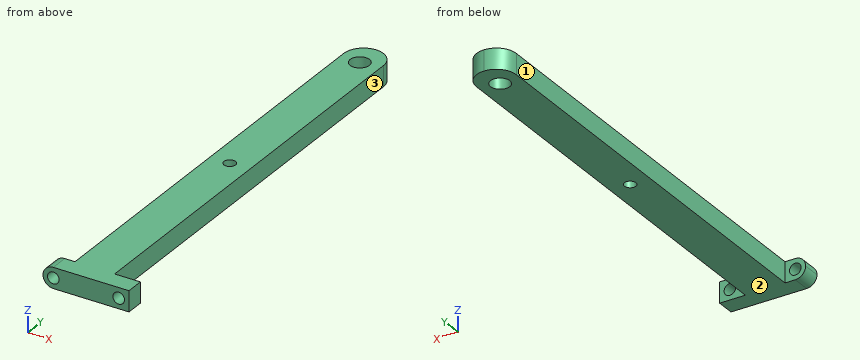
Autodesk Inventor part; units mm, degrees
ref_plane "YZ Plane" through (0, 0, 0) normal (1, 0, 0) x (0, 1, 0)
ref_plane "XZ Plane" through (0, 0, 0) normal (0, 1, 0) x (-1, 0, 0)
ref_plane "XY Plane" through (0, 0, 0) normal (0, 0, 1) x (1, 0, 0)
sketch "Sketch1" plane through (0, 0, 0) normal (0, 0, 1) x (1, 0, 0)
  line L0 (-15.4, 0) -> (0, 0)
  line L1 (0, 0) -> (0, 180)
  line L2 (0, 180) -> (-15.4, 180)
  line L3 (-15.4, 180) -> (-15.4, 0)
  point P0 (0, 0)
  point P1 (-7.7, 170)
  dimension "d0" = 15.4
  dimension "d1" = 180
  dimension "d2" = 0
  dimension "d3" = 0
  dimension "d4" = 7.7
  dimension "d5" = 170
extrude "Extrusion1" add sketch "Sketch1" along normal blind 8
hole "Hole1" at (-7.7, 170, 0) direction (0, 0, 1) diameter 7.525 end through all
sketch "Sketch2" plane through (0, 0, 0) normal (1, 0, 0) x (0, 0, -1)
  point P0 (0, 0)
sketch "Sketch5" plane through (0, 0, 0) normal (0, 0, -1) x (-1, 0, 0)
  line L0 (15.4, 180) -> (15.4, 0)
  line L1 (15.4, 0) -> (0, 0)
  point P0 (7.7, 90)
  dimension "d27" = 7.7
  dimension "d28" = 90
full round fillet "Full Round Fillet1" first side at (0, 60, 2.6667) centre faces at (-5.1333, 180, 2.6667) second side at (-15.4, 120, 2.6667)
hole "Hole3" at (-7.7, 90, 0) direction (0, 0, 1) diameter 4.5 end through all
sketch "Sketch6" plane through (0, 0, 8) normal (1, 0, 0) x (0, 0, -1)
  line L0 (0, 172.3) -> (0, 0)
  line L1 (8, 172.3) -> (8, 0)
  line L2 (0, 0) -> (8, 0)
  line L3 (8, 0) -> (8, 7)
  line L4 (8, 7) -> (0, 7)
  line L5 (0, 7) -> (0, 0)
  point P0 (8, 0)
  point P1 (0, 7)
  dimension "d36" = 7
extrude "Extrusion3" add sketch "Sketch6" along normal blind 10
sketch "Sketch7" plane through (0, 7, 8) normal (0, 1, 0) x (1, 0, 0)
  line L0 (0, 8) -> (10, 8)
  line L1 (10, 8) -> (10, 0)
  point P0 (6, 4)
  dimension "d39" = 4
  dimension "d40" = 4
hole "Hole4" at (6, 7, 4) direction (0, -1, 0) diameter 4.5 end through all
sketch "Sketch8" plane through (-15.4, 0, 0) normal (-1, 0, 0) x (0, 0, 1)
  point P0 (0, 0)
sketch "Sketch9" plane through (-15.4, 0, 0) normal (-1, 0, 0) x (0, 0, 1)
  line L0 (0, 0) -> (8, 0)
  line L1 (8, 7) -> (8, 172.3)
  line L2 (0, 0) -> (8, 0)
  line L3 (8, 0) -> (8, 7)
  line L4 (8, 7) -> (0, 7)
  line L5 (0, 7) -> (0, 0)
extrude "Extrusion4" add sketch "Sketch9" along normal blind 8
sketch "Sketch10" plane through (-15.4, 7, 8) normal (0, 1, 0) x (1, 0, 0)
  line L0 (-8, 0) -> (-8, 8)
  line L1 (0, 8) -> (-8, 8)
  line L2 (0, 8) -> (0, 0)
  point P0 (15.4, 8)
  point P1 (-4, 4)
  dimension "d51" = 4
  dimension "d59" = 4
hole "Hole5" at (-19.4, 7, 4) direction (0, -1, 0) diameter 4.5 end through all
full round fillet "Full Round Fillet2" first side at (-7.7, 33.9167, 8) centre faces at (-23.4, 2.3333, 2.6667) second side at (-7.7, 33.9167, 0)
properties part number "Slide Strut"
Work out the finished part from the listing and answer in its coordinate system (mm). Face numbers are marked on the shaded views. A direction names the side the tool comes from. Give positions to 0.01 mm unless a question says otherwise; leave off trailing zeros. Order: outer loops, then holes, each group sorted by start corner. A loop starts at its lowest first (then second) coordinate and runs counter-clockwise, first axis right, second up. Notation, with made-up numbers: (67.25, 80.25) - (106.25, 80.25) arc R25 cw to (106.25, 112.25) - close; hole circle Ø1 at (-10.5, -8). An arc over 180 degrees is marked (long way). One line per item, written item: value. Start each with the question number.
1. Consider line 1 (X direction, y = 3.5, z = 4); line 2 (Y direction, x = -7.7, z = 3.5); line 3 (Y direction, x = -6.5, z = 1.25). Determine where each line is inside the solid, lowest interval first.
2. Section A-A, the plane y = 90 is taken. Write down the section's boundary in (x, z).
3. Each of these flat-tipped pins is pushed along its axis until it touches: pin 1 Ø4 at (x, z) = (-19.4, 4) entering from +Y; pin 2 Ø4 at (y, z) = (58, 6) entering from -X; pin 3 Ø2.5 at (x, z) = (-17.5, 3) entering from +Y; pin 4 Ø4 at (y, z) = (100.5, 2) entering from +X. Where does it stop, or does it pass through?
4. Which of the six approach directions +Z, -Z, +X, -X, +Y, -Y give full straight-line access (tool end or side, diameter ignored) to the marked faces 1, 2 and 3?
5. Section B-B, the plane x = 6 is taken. Write down the section's boundary in (y, z), then the cut area to 3 significant figures.
Filled sheet:
1. line 1: -23.4 to -21.65, -17.15 to 3.75, 8.25 to 10
1. line 2: 0 to 87.75, 92.25 to 166.24, 173.76 to 180
1. line 3: 0 to 88.1, 91.9 to 166.43, 173.57 to 179.91
2. outline: (-15.4, 0) - (-9.95, 0) - (-9.95, 8) - (-15.4, 8) - close; (-5.45, 0) - (0, 0) - (0, 8) - (-5.45, 8) - close
3. pin 1: through
3. pin 2: x = -15.4
3. pin 3: y = 7
3. pin 4: x = 0
4. face 1: +Z, -Z, -X, +Y
4. face 2: -Z, +X, -X, +Y, -Y
4. face 3: +Z, -Z, +X, +Y
5. outline: (0, 0) - (7, 0) - (7, 1.75) - (0, 1.75) - close; (0, 6.25) - (7, 6.25) - (7, 8) - (0, 8) - close
5. area: 24.5 mm²
